```python
from build123d import *

# Parameters (mm, degrees)
F0_R     = 4.7625
F0_R_2   = 1.5875
F1_DEPTH = 6.35
F2_COUNT = 15
F3_R     = 4.7625
F3_R_2   = 3.175
F3_R_3   = 1.5875
F4_DEPTH = 6.35
F5_R     = 5.08
F5_R_2   = 3.175
F6_DEPTH = 1.016
F7_R     = 1.01599
F8_SIZE  = 0.254


# Not quite as in the source:
# - a fillet or chamfer is up to 0.001 mm smaller than in the source, because OpenCascade refuses the exact size


with BuildPart() as f1:
    # F0 (on Top) → F1 (new body)
    with BuildSketch(Plane.XY):
        with BuildLine():
            ThreePointArc((-1.9696004156, 12.5463410683), (-8.2545767524, -9.6515264409), (12.7, 0))
            ThreePointArc((12.7, 0), (9.6515264409, 8.2545767524), (1.9696004156, 12.5463410683))
            ThreePointArc((1.9696004156, 12.5463410683), (0, 12.7), (-1.9696004156, 12.5463410683))
        make_face()
        Circle(F0_R, mode=Mode.SUBTRACT)
        with BuildLine():
            ThreePointArc((-1.9696004156, 12.5463410683), (0, 12.7), (1.9696004156, 12.5463410683))
            ThreePointArc((1.9696004156, 12.5463410683), (1.4239736696, 14.2389394562), (0.6924577744, 15.8598905176))
            ThreePointArc((0.6924577744, 15.8598905176), (0, 15.875), (-0.6924577744, 15.8598905176))
            ThreePointArc((-0.6924577744, 15.8598905176), (-1.4239736696, 14.2389394562), (-1.9696004156, 12.5463410683))
        make_face()
        Circle(F0_R)
        Circle(F0_R_2, mode=Mode.SUBTRACT)
    extrude(amount=F1_DEPTH)

    # F2: F1 ×15 about axis
    f2_axis = Axis((0, 0, 0), (0, 0, -1))


with BuildPart() as f1_1:
    add(f1.part)
    for i in range(1, F2_COUNT):
        add(f1.part.rotate(f2_axis, i * 360 / F2_COUNT))

    # F3 (on face) → F4 (join)
    with BuildSketch(Plane.XY.offset(6.35)):
        with BuildLine():
            ThreePointArc((6.3411298165, -0.3355184801), (6.3477820668, -0.1678178556), (6.35, 0))
            ThreePointArc((6.35, 0), (6.222203729, 1.2675491134), (5.8439588173, 2.4840783686))
            ThreePointArc((5.8439588173, 2.4840783686), (5.499261314, 3.175), (5.0732543809, 3.8189776102))
            ThreePointArc((5.0732543809, 3.8189776102), (4.0817013215, 4.8643822138), (2.879997381, 5.6593387498))
            ThreePointArc((2.879997381, 5.6593387498), (2.1718279101, 5.967048142), (1.4315468375, 6.1865316335))
            ThreePointArc((1.4315468375, 6.1865316335), (0, 6.35), (-1.4315468375, 6.1865316335))
            ThreePointArc((-1.4315468375, 6.1865316335), (-2.1718279101, 5.967048142), (-2.879997381, 5.6593387498))
            ThreePointArc((-2.879997381, 5.6593387498), (-4.0817013215, 4.8643822138), (-5.0732543809, 3.8189776102))
            ThreePointArc((-5.0732543809, 3.8189776102), (-5.499261314, 3.175), (-5.8439588173, 2.4840783686))
            ThreePointArc((-5.8439588173, 2.4840783686), (-6.2535292316, 1.1026659282), (-6.3411298165, -0.3355184801))
            ThreePointArc((-6.3411298165, -0.3355184801), (-6.2535292316, -1.1026659282), (-6.0734669747, -1.8535098888))
            ThreePointArc((-6.0734669747, -1.8535098888), (-5.499261314, -3.175), (-4.6419201372, -4.3330217447))
            ThreePointArc((-4.6419201372, -4.3330217447), (-4.0817013215, -4.8643822138), (-3.4611324355, -5.3238202697))
            ThreePointArc((-3.4611324355, -5.3238202697), (-2.1718279101, -5.967048142), (-0.7707044365, -6.3030559788))
            ThreePointArc((-0.7707044365, -6.3030559788), (0, -6.35), (0.7707044365, -6.3030559788))
            ThreePointArc((0.7707044365, -6.3030559788), (2.1718279101, -5.967048142), (3.4611324355, -5.3238202697))
            ThreePointArc((3.4611324355, -5.3238202697), (4.0817013215, -4.8643822138), (4.6419201372, -4.3330217447))
            ThreePointArc((4.6419201372, -4.3330217447), (5.499261314, -3.175), (6.0734669747, -1.8535098888))
            ThreePointArc((6.0734669747, -1.8535098888), (6.2535292316, -1.1026659282), (6.3411298165, -0.3355184801))
        make_face()
        Circle(F3_R, mode=Mode.SUBTRACT)
        with BuildLine():
            ThreePointArc((5.8439588173, 2.4840783686), (6.222203729, 1.2675491134), (6.35, 0))
            ThreePointArc((6.35, 0), (6.3477820668, -0.1678178556), (6.3411298165, -0.3355184801))
            ThreePointArc((6.3411298165, -0.3355184801), (7.9650557648, 0.3109444224), (9.4435123046, 1.2432619809))
            ThreePointArc((9.4435123046, 1.2432619809), (9.3802938474, 1.6539988923), (9.2992194678, 2.0615873228))
            ThreePointArc((9.2992194678, 2.0615873228), (7.5910533822, 2.4320173351), (5.8439588173, 2.4840783686))
        make_face()
        with BuildLine():
            ThreePointArc((2.879997381, 5.6593387498), (4.0817013215, 4.8643822138), (5.0732543809, 3.8189776102))
            ThreePointArc((5.0732543809, 3.8189776102), (5.9017154857, 5.358036403), (6.4349967275, 7.0225666331))
            ThreePointArc((6.4349967275, 7.0225666331), (6.1225519823, 7.2965733207), (5.7984526113, 7.5566905663))
            ThreePointArc((5.7984526113, 7.5566905663), (4.2518136514, 6.7424684237), (2.879997381, 5.6593387498))
        make_face()
        with BuildLine():
            ThreePointArc((8.448778186, -4.3981555411), (7.3783548704, -3.0164016935), (6.0734669747, -1.8535098888))
            ThreePointArc((6.0734669747, -1.8535098888), (5.499261314, -3.175), (4.6419201372, -4.3330217447))
            ThreePointArc((4.6419201372, -4.3330217447), (6.3014579298, -4.8816419092), (8.0333035214, -5.1177787695))
            ThreePointArc((8.0333035214, -5.1177787695), (8.248891971, -4.7625), (8.448778186, -4.3981555411))
        make_face()
        with BuildLine():
            ThreePointArc((-1.4315468375, 6.1865316335), (0, 6.35), (1.4315468375, 6.1865316335))
            ThreePointArc((1.4315468375, 6.1865316335), (1.0768969406, 7.8980436026), (0.4154746647, 9.5159343106))
            ThreePointArc((0.4154746647, 9.5159343106), (0, 9.525), (-0.4154746647, 9.5159343106))
            ThreePointArc((-0.4154746647, 9.5159343106), (-1.0768969406, 7.8980436026), (-1.4315468375, 6.1865316335))
        make_face()
        with BuildLine():
            ThreePointArc((3.6450596933, -8.7999525472), (3.7132421134, -7.0534128461), (3.4611324355, -5.3238202697))
            ThreePointArc((3.4611324355, -5.3238202697), (2.1718279101, -5.967048142), (0.7707044365, -6.3030559788))
            ThreePointArc((0.7707044365, -6.3030559788), (1.6893378965, -7.790053738), (2.8642227403, -9.0841539559))
            ThreePointArc((2.8642227403, -9.0841539559), (3.2577418652, -8.950572213), (3.6450596933, -8.7999525472))
        make_face()
        with BuildLine():
            ThreePointArc((-5.0732543809, 3.8189776102), (-4.0817013215, 4.8643822138), (-2.879997381, 5.6593387498))
            ThreePointArc((-2.879997381, 5.6593387498), (-4.2518136514, 6.7424684237), (-5.7984526113, 7.5566905663))
            ThreePointArc((-5.7984526113, 7.5566905663), (-6.1225519823, 7.2965733207), (-6.4349967275, 7.0225666331))
            ThreePointArc((-6.4349967275, 7.0225666331), (-5.9017154857, 5.358036403), (-5.0732543809, 3.8189776102))
        make_face()
        with BuildLine():
            ThreePointArc((-2.8642227403, -9.0841539559), (-1.6893378965, -7.790053738), (-0.7707044365, -6.3030559788))
            ThreePointArc((-0.7707044365, -6.3030559788), (-2.1718279101, -5.967048142), (-3.4611324355, -5.3238202697))
            ThreePointArc((-3.4611324355, -5.3238202697), (-3.7132421134, -7.0534128461), (-3.6450596933, -8.7999525472))
            ThreePointArc((-3.6450596933, -8.7999525472), (-3.2577418652, -8.950572213), (-2.8642227403, -9.0841539559))
        make_face()
        with BuildLine():
            ThreePointArc((-6.3411298165, -0.3355184801), (-6.2535292316, 1.1026659282), (-5.8439588173, 2.4840783686))
            ThreePointArc((-5.8439588173, 2.4840783686), (-7.5910533822, 2.4320173351), (-9.2992194678, 2.0615873228))
            ThreePointArc((-9.2992194678, 2.0615873228), (-9.3802938474, 1.6539988923), (-9.4435123046, 1.2432619809))
            ThreePointArc((-9.4435123046, 1.2432619809), (-7.9650557648, 0.3109444224), (-6.3411298165, -0.3355184801))
        make_face()
        with BuildLine():
            ThreePointArc((-8.0333035214, -5.1177787695), (-6.3014579298, -4.8816419092), (-4.6419201372, -4.3330217447))
            ThreePointArc((-4.6419201372, -4.3330217447), (-5.499261314, -3.175), (-6.0734669747, -1.8535098888))
            ThreePointArc((-6.0734669747, -1.8535098888), (-7.3783548704, -3.0164016935), (-8.448778186, -4.3981555411))
            ThreePointArc((-8.448778186, -4.3981555411), (-8.248891971, -4.7625), (-8.0333035214, -5.1177787695))
        make_face()
        Circle(F3_R)
        Circle(F3_R_2, mode=Mode.SUBTRACT)
        Circle(F3_R_2)
        Circle(F3_R_3, mode=Mode.SUBTRACT)
    extrude(amount=F4_DEPTH)

    # F5 (on face) → F6 (cut)
    with BuildSketch(Plane.XY.offset(12.7)):
        Circle(F5_R)
        Circle(F5_R_2, mode=Mode.SUBTRACT)
    extrude(amount=-F6_DEPTH, mode=Mode.SUBTRACT)

    # F7 (radius 1.016 in the source; OpenCascade refuses exactly that, so slightly less here)
    f7_edges = [f1_1.edges().sort_by_distance(p)[0] for p in [
        (-5.08, 0, 11.684),
    ]]
    fillet(f7_edges, radius=F7_R)

    # F8
    f8_edges = [f1_1.edges().sort_by_distance(p)[0] for p in [
        (-1.5875, 0, 12.7),
        (-3.175, 0, 12.7),
    ]]
    chamfer(f8_edges, length=F8_SIZE)


solid = f1_1.part
```
For this review, take the finished solid that the model builds, in its own axes (mm). A direction names the side the tool comes from. Coordinates: 2 decimals unless noted, no trailing zeros. Loops run counter-clockwise (first coordinate to the right, second up) from the corner with the lowest first, then second, coordinate; pieces in that order, holes last.
1. Mouldability with a two-part tool opening along X and no side actions: class faces 1 (the cylindrical face through (11.5, 8.4, 3.1)), 2 (the cylindrical face through (-15.1, 4.9, 3.1)), 3 (the cylindrical face through (-1.58, -14.24, 3.13)) as +X half, -X half, draft (parallel to the pull), parting line (faces both ways), or undercut.
2. Insertion check: P1, Ø3, axis at x = 3, z = 7.5, coming from the -Y side; P2, Ø1, axis at y = 9.5, z = 9.5, coming from the +X side; P3, Ø5, axis at y = -9, z = 7.5, coming from the -X side; P4, Ø1, axis at x = 11, y = -8, coming from the +Z side. Each pin has a flat end and moves straight along its axis. Give the tip position at first contact, or say it passes through.
3. Add section B-B, the plane y = 8. Give the boundary of the cut face in (x, z), then the cut area to 3 significant figures.
4. For line 1 (X direction, y = 6.5, z = 9.75); line 2 (Z direction, x = 8.5, y = 2.5); line 3 (Z direction, x = -3, y = -2.5), list the stretches that pass through material, from the lowest coordinate up.
5. For faces 4 (the cylindrical face through (14.332, -0.084, 3.131)), 5 (the cylindrical face through (-2.16, 5.97, 9.48)), 6 (the cylindrical face through (-0.01, -6.35, 9.48)), list the 3-axis set-ups (+Z, -Z, +X, -X, +Y, -Y) from which the entire face can be reached by the end or side of a thin tool; tool diameter is ignored.
Result:
1. face 1: +X half
1. face 2: -X half
1. face 3: undercut
2. P1: stops at y = -15.66
2. P2: stops at x = 0.66
2. P3: stops at x = -14.08
2. P4: stops at z = 6.35
3. outline: (-11.29, 0) - (11.29, 0) - (11.29, 6.35) - (1.05, 6.35) - (1.05, 12.7) - (-1.05, 12.7) - (-1.05, 6.35) - (-11.29, 6.35) - close
3. area: 157 mm2
4. line 1: x = -6.3 to -3.9, -1.39 to 1.39, 3.9 to 6.3
4. line 2: z = 0 to 6.35
4. line 3: z = 0 to 11.68
5. face 4: +Z, -Z, +X
5. face 5: +Z, +Y
5. face 6: +Z, -Y
